Could you check a few things on this model? Use its own coordinates, in mm. A direction names the side the tool comes from. Give positions to 0.01 mm unless a question says otherwise; leave off trailing zeros. One line per item, written item: value.
```python
from build123d import *

# Parameters (mm, degrees)
BOSS_EXTRUDE1_DEPTH = 5
BOSS_EXTRUDE3_DEPTH = 20
FILLET5_R           = 30
FILLET6_R           = 33
FILLET4_R           = 5
REVOLVE3_ANGLE      = 90
BOSS_EXTRUDE4_DEPTH = 20
CUT_EXTRUDE1_REACH  = 577.05
SKETCH10_R          = 7.5
FILLET7_R           = 3


with BuildPart() as part:
    # Sketch1 → Boss-Extrude1 (new body)
    with BuildSketch(Plane(origin=(0, 0, 0), x_dir=(1, 0, 0), z_dir=(0, 1, 0))):
        Polygon((-165, 270), (-165, -270), (0, -270), (0, -250), (-145, -250), (-145, 250), (0, 250), (0, 270), align=None)
    extrude(amount=BOSS_EXTRUDE1_DEPTH)

    # Sketch7 → Boss-Extrude3 (add)
    with BuildSketch(Plane(origin=(0, 5, 0), x_dir=(1, 0, 0), z_dir=(0, 1, 0))):
        Polygon((0, 253), (-148, 253), (-148, -253), (0, -253), (0, -250), (-145, -250), (-145, 250), (0, 250), align=None)
    extrude(amount=BOSS_EXTRUDE3_DEPTH)

    # Fillet5
    fillet5_edges = [part.edges().sort_by_distance(p)[0] for p in [
        (-145, 12.5, -250),
        (-145, 12.5, 250),
    ]]
    fillet(fillet5_edges, radius=FILLET5_R)

    # Fillet6
    fillet6_edges = [part.edges().sort_by_distance(p)[0] for p in [
        (-148, 15, -253),
        (-148, 15, 253),
    ]]
    fillet(fillet6_edges, radius=FILLET6_R)

    # Fillet4
    fillet4_edges = [part.edges().sort_by_distance(p)[0] for p in [
        (-165, 2.5, 270),
        (-165, 2.5, -270),
    ]]
    fillet(fillet4_edges, radius=FILLET4_R)

    # Sketch8 → Revolve3 (revolve)
    with BuildSketch(Plane(origin=(0, 25, 0), x_dir=(1, 0, 0), z_dir=(0, 1, 0))):
        with BuildLine():
            Line((0, 253), (-115, 253))
            ThreePointArc((-115, 253), (-138.334523779, 243.334523779), (-148, 220))
            Line((-148, 220), (-148, -220))
            ThreePointArc((-148, -220), (-138.334523779, -243.334523779), (-115, -253))
            Line((-115, -253), (0, -253))
            Line((0, -253), (0, -250))
            Line((0, -250), (-115, -250))
            ThreePointArc((-115, -250), (-136.213203436, -241.213203436), (-145, -220))
            Line((-145, -220), (-145, 220))
            ThreePointArc((-145, 220), (-136.213203436, 241.213203436), (-115, 250))
            Line((-115, 250), (0, 250))
            Line((0, 250), (0, 253))
        make_face()
    revolve(axis=Axis((0, 25, -250), (0, 0, -1)), revolution_arc=REVOLVE3_ANGLE)

    # Sketch9 → Boss-Extrude4 (add)
    with BuildSketch(Plane(origin=(0, 0, 0), x_dir=(0, 0, -1), z_dir=(1, 0, 0))):
        with BuildLine():
            Line((253, 25), (253, 140))
            ThreePointArc((253, 140), (243.334523779, 163.334523779), (220, 173))
            Line((220, 173), (-220, 173))
            ThreePointArc((-220, 173), (-243.334523779, 163.334523779), (-253, 140))
            Line((-253, 140), (-253, 25))
            Line((-253, 25), (-253, 5))
            Line((-253, 5), (-270, 5))
            Line((-270, 5), (-270, 0))
            Line((-270, 0), (-250, 0))
            Line((-250, 0), (-250, 25))
            Line((-250, 25), (-250, 140))
            ThreePointArc((-250, 140), (-241.213203436, 161.213203436), (-220, 170))
            Line((-220, 170), (220, 170))
            ThreePointArc((220, 170), (241.213203436, 161.213203436), (250, 140))
            Line((250, 140), (250, 25))
            Line((250, 25), (250, 0))
            Line((250, 0), (270, 0))
            Line((270, 0), (270, 5))
            Line((270, 5), (253, 5))
            Line((253, 5), (253, 25))
        make_face()
    extrude(amount=BOSS_EXTRUDE4_DEPTH)

    # Cut-Extrude1: up to this face of the body (flat: up to its plane)
    cut_extrude1_end = Plane(part.part.faces().sort_by_distance((-39.787657223, 64.787657223, -253))[0])
    # Sketch10 → Cut-Extrude1 (cut, up to the picked face)
    with BuildSketch(Plane.XY.offset(253), mode=Mode.PRIVATE) as cut_extrude1_sk1:
        with Locations((0, 25)):
            Circle(SKETCH10_R)
    cut_extrude1_tool1 = split(extrude(cut_extrude1_sk1.sketch, amount=-CUT_EXTRUDE1_REACH, mode=Mode.PRIVATE), bisect_by=cut_extrude1_end, keep=Keep.BOTH, mode=Mode.PRIVATE)
    add(cut_extrude1_tool1.solids().sort_by(Axis((0, 25, 253), (0, 0, -1)))[0], mode=Mode.SUBTRACT)

    # Fillet7
    fillet7_edges = [part.edges().sort_by_distance(p)[0] for p in [
        (20, 72.5, -253),
        (20, 163.334523779, -243.334523779),
        (20, 173, 0),
        (20, 163.334523779, 243.334523779),
        (20, 72.5, 253),
    ]]
    fillet(fillet7_edges, radius=FILLET7_R - 0.0001)  # a hair under: the kernel refuses the full size


solid = part.part
```
1) I'm going to push flat-ended pins straight in: pin 1 (6 mm diameter, centred on x = -136.5, z = -78.5, fed in from +Y); pin 2 (19.5 mm diameter, centred on x = 0, y = 25, fed in from +Z); pin 3 (1.5 mm diameter, centred on y = 117.5, z = -110.5, fed in from +X). Where does each tip first touch, or does it pass through?
Outcome:
pin 1: stops at y = 88.89
pin 2: stops at z = 253
pin 3: stops at x = -111.04
2) We'd pull the mould along Z, two halves only. Please class faces 1 (the face through (-48, 71, -250)), 2 (the face through (8.381, 163.59, 243.077)), 3 (the face through (8, 173, -3)): pulls with the +Z half, pulls with the -Z half, needs draft (parallel to the pull), parting line crosses it, or undercut.
Outcome:
face 1: undercut
face 2: pulls with the +Z half
face 3: needs draft
3) On a 3-axis mill with a long thin cutter (end or side, diameter ignored), from which of +Z, -Z, +X, -X, +Y, -Y can I reach the whole of each face in a straight line? I mean faces 4 (the face through (-145, 12, 3)), 5 (the face through (-138.077, 15.14, 243.59)), 6 (the face through (-138.59, 15.14, -243.077)), 7 (the face through (-50, 72, -253)). Say none if no direction works.
Outcome:
face 4: +X, -Y
face 5: +Z, -X, +Y
face 6: -Z, -X, +Y
face 7: -Z, +X, -X, +Y
4) Please list where these lines run through material, in increasing order: L1, parallel to Z at x = -65.5, y = 66.5; L2, parallel to X at y = 29, z = -84.5; L3, parallel to Y at x = -33, z = -195.5. Write a range as from..to.
Outcome:
L1: z = -253..-250, 250..253
L2: x = -147.95..-144.94
L3: y = 166.19..169.27
